Check sheet for the modelled part. Datum: model origin and axes. Units: mm. Face numbers are marked on the shaded views. Give positions to 0.01 mm unless a question says otherwise; leave off trailing zeros. Order: outer loops, then holes, each group sorted by start corner. A loop starts at its lowest first (then second) coordinate and runs counter-clockwise, first axis right, second up. Notation, with made-up numbers: (63, 40) - (85, 40) arc R7 ccw to (85, 47) - close; hole circle Ø7 at (-5, 0). An arc over 180 degrees is marked (long way). Answer in a Markdown table with one row per item.
from build123d import *

# Parameters (mm, degrees)
SKETCH1_R           = 1.75
BOSS_EXTRUDE2_DEPTH = 3
CUT_EXTRUDE5_DEPTH  = 117.344085899


with BuildPart() as part:
    # Sketch1 → Boss-Extrude2 (new body)
    # profile 1 of 6: a face of its own
    with BuildSketch(Plane.XY):
        with BuildLine():
            Line((-61.518289963, 44.547727215), (-78.684996473, 61.714433725))
            ThreePointArc((-78.684996473, 61.714433725), (-82.079566173, 51.162002537), (-75.485462345, 42.251632055))
            ThreePointArc((-75.485462345, 42.251632055), (-69.588581896, 41.003233411), (-63.818207412, 42.745208303))
            ThreePointArc((-63.818207412, 42.745208303), (-63.605961831, 42.89146595), (-63.383207651, 43.021158129))
            ThreePointArc((-63.383207651, 43.021158129), (-62.41276888, 43.738044879), (-61.518289963, 44.547727215))
        make_face()
        with Locations((-75.306872196, 51.265241636)):
            Circle(SKETCH1_R, mode=Mode.SUBTRACT)
    # profile 2 of 6: a face of its own
    with BuildSketch(Plane.XY):
        with BuildLine():
            ThreePointArc((-63.818207412, 42.745208303), (-69.588581896, 41.003233411), (-75.485462345, 42.251632055))
            ThreePointArc((-75.485462345, 42.251632055), (-66.626510988, 39.720558383), (-58.255022397, 43.568354094))
            ThreePointArc((-58.255022397, 43.568354094), (-59.291136488, 43.01863263), (-60.457290906, 43.144370333))
            ThreePointArc((-60.457290906, 43.144370333), (-61.934255267, 43.415364041), (-63.383207651, 43.021158129))
            ThreePointArc((-63.383207651, 43.021158129), (-63.599243517, 42.880875383), (-63.818207412, 42.745208303))
        make_face()
    # profile 3 of 6: a face of its own
    with BuildSketch(Plane.XY):
        with BuildLine():
            Line((-53.033008589, 53.033008589), (-61.518289963, 44.547727215))
            ThreePointArc((-61.518289963, 44.547727215), (-62.41276888, 43.738044879), (-63.383207651, 43.021158129))
            ThreePointArc((-63.383207651, 43.021158129), (-61.934255267, 43.415364041), (-60.457290906, 43.144370333))
            ThreePointArc((-60.457290906, 43.144370333), (-59.291136488, 43.01863263), (-58.255022397, 43.568354094))
            Line((-58.255022397, 43.568354094), (-50.911688245, 50.911688245))
            Line((-50.911688245, 50.911688245), (-53.033008589, 53.033008589))
        make_face()
    # profile 4 of 6: a face of its own
    with BuildSketch(Plane.XY):
        with BuildLine():
            Line((-44.547727215, 61.518289963), (-53.033008589, 53.033008589))
            Line((-53.033008589, 53.033008589), (-50.911688245, 50.911688245))
            Line((-50.911688245, 50.911688245), (-43.568354094, 58.255022397))
            ThreePointArc((-43.568354094, 58.255022397), (-43.01863263, 59.291136488), (-43.144370333, 60.457290906))
            ThreePointArc((-43.144370333, 60.457290906), (-43.415364041, 61.934255267), (-43.021158129, 63.383207651))
            ThreePointArc((-43.021158129, 63.383207651), (-43.738044879, 62.41276888), (-44.547727215, 61.518289963))
        make_face()
    # profile 5 of 6: a face of its own
    with BuildSketch(Plane.XY):
        with BuildLine():
            ThreePointArc((-42.745208303, 63.818207412), (-42.880875383, 63.599243517), (-43.021158129, 63.383207651))
            ThreePointArc((-43.021158129, 63.383207651), (-43.415364041, 61.934255267), (-43.144370333, 60.457290906))
            ThreePointArc((-43.144370333, 60.457290906), (-43.01863263, 59.291136488), (-43.568354094, 58.255022397))
            ThreePointArc((-43.568354094, 58.255022397), (-39.720558383, 66.626510988), (-42.251632055, 75.485462345))
            ThreePointArc((-42.251632055, 75.485462345), (-41.003233411, 69.588581896), (-42.745208303, 63.818207412))
        make_face()
    # profile 6 of 6: a face of its own
    with BuildSketch(Plane.XY):
        with BuildLine():
            Line((-61.714433725, 78.684996473), (-44.547727215, 61.518289963))
            ThreePointArc((-44.547727215, 61.518289963), (-43.738044879, 62.41276888), (-43.021158129, 63.383207651))
            ThreePointArc((-43.021158129, 63.383207651), (-42.89146595, 63.605961831), (-42.745208303, 63.818207412))
            ThreePointArc((-42.745208303, 63.818207412), (-41.003233411, 69.588581896), (-42.251632055, 75.485462345))
            ThreePointArc((-42.251632055, 75.485462345), (-51.162002537, 82.079566173), (-61.714433725, 78.684996473))
        make_face()
        with Locations((-51.265241636, 75.306872196)):
            Circle(SKETCH1_R, mode=Mode.SUBTRACT)
    extrude(amount=BOSS_EXTRUDE2_DEPTH)

    # Sketch2 → Cut-Extrude5 (cut, through all)
    with BuildSketch(Plane.XY.offset(3)):
        with BuildLine():
            Line((-87.146030282, 55.882108481), (-82.002155393, 50.738233593))
            ThreePointArc((-82.002155393, 50.738233593), (-81.721300187, 56.642700912), (-78.684996473, 61.714433725))
            Line((-78.684996473, 61.714433725), (-74.855475867, 57.884913119))
            Line((-74.855475867, 57.884913119), (-73.595511338, 59.144877648))
            Line((-73.595511338, 59.144877648), (-82.002155393, 67.551521704))
            Line((-82.002155393, 67.551521704), (-87.146030282, 55.882108481))
        make_face()
        with BuildLine():
            ThreePointArc((-78.684996473, 61.714433725), (-81.721300187, 56.642700912), (-82.002155393, 50.738233593))
            Line((-82.002155393, 50.738233593), (-74.855475867, 57.884913119))
            Line((-74.855475867, 57.884913119), (-78.684996473, 61.714433725))
        make_face()
        with BuildLine():
            Line((-71.077925903, 40.135754876), (-82.002155393, 50.738233593))
            ThreePointArc((-82.002155393, 50.738233593), (-79.729344323, 45.738159691), (-75.485462345, 42.251632055))
            ThreePointArc((-75.485462345, 42.251632055), (-73.379988253, 40.988939163), (-71.077925903, 40.135754876))
        make_face()
        with BuildLine():
            ThreePointArc((-75.485462345, 42.251632055), (-79.729344323, 45.738159691), (-82.002155393, 50.738233593))
            Line((-82.002155393, 50.738233593), (-82.002155393, 40.135754876))
            Line((-82.002155393, 40.135754876), (-71.077925903, 40.135754876))
            ThreePointArc((-71.077925903, 40.135754876), (-73.379988253, 40.988939163), (-75.485462345, 42.251632055))
        make_face()
        with BuildLine():
            ThreePointArc((-61.714433725, 78.684996473), (-56.642700912, 81.721300187), (-50.738233593, 82.002155393))
            Line((-50.738233593, 82.002155393), (-55.882108481, 87.146030282))
            Line((-55.882108481, 87.146030282), (-67.551521704, 82.002155393))
            Line((-67.551521704, 82.002155393), (-59.144877648, 73.595511338))
            Line((-59.144877648, 73.595511338), (-57.884913119, 74.855475867))
            Line((-57.884913119, 74.855475867), (-61.714433725, 78.684996473))
        make_face()
        with BuildLine():
            Line((-57.884913119, 74.855475867), (-50.738233593, 82.002155393))
            ThreePointArc((-50.738233593, 82.002155393), (-56.642700912, 81.721300187), (-61.714433725, 78.684996473))
            Line((-61.714433725, 78.684996473), (-57.884913119, 74.855475867))
        make_face()
        with BuildLine():
            ThreePointArc((-42.251632055, 75.485462345), (-45.738159691, 79.729344323), (-50.738233593, 82.002155393))
            Line((-50.738233593, 82.002155393), (-40.135754876, 71.077925903))
            ThreePointArc((-40.135754876, 71.077925903), (-40.988939163, 73.379988253), (-42.251632055, 75.485462345))
        make_face()
        with BuildLine():
            Line((-40.135754876, 82.002155393), (-50.738233593, 82.002155393))
            ThreePointArc((-50.738233593, 82.002155393), (-45.738159691, 79.729344323), (-42.251632055, 75.485462345))
            ThreePointArc((-42.251632055, 75.485462345), (-40.988939163, 73.379988253), (-40.135754876, 71.077925903))
            Line((-40.135754876, 71.077925903), (-40.135754876, 82.002155393))
        make_face()
    extrude(amount=-CUT_EXTRUDE5_DEPTH, mode=Mode.SUBTRACT)


solid = part.part
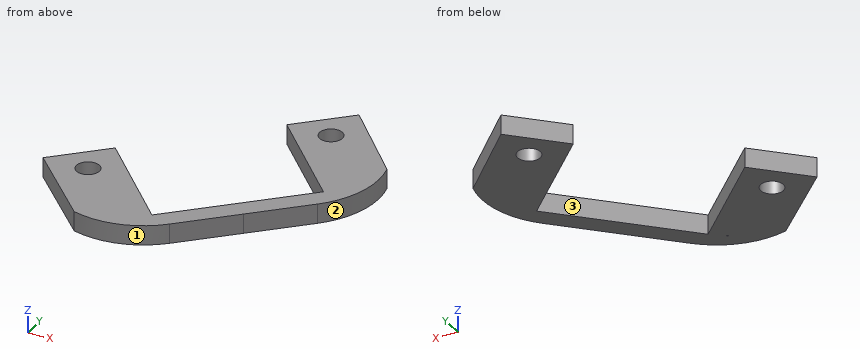
(1) Cross-section at C-C, the plane y = 76.5. Record the cut outline in (x, z), then the cut area to 3 significant figures.
Geometry says:
| item | result |
|---|---|
| outline | (-56.24, 0) - (-52.55, 0) - (-52.55, 3) - (-56.24, 3) - close; (-49.99, 0) - (-45.4, 0) - (-45.4, 3) - (-49.99, 3) - close |
| area | 24.8 mm² |
(2) Cross-section at B-B, the plane y = 50. Record the cut outline in (x, z), then the cut area to 3 significant figures.
Geometry says:
| item | result |
|---|---|
| outline | (-81.24, 0) - (-76.52, 0) - (-76.52, 3) - (-81.24, 3) - close; (-74.1, 0) - (-66.97, 0) - (-66.97, 3) - (-74.1, 3) - close; (-56.07, 0) - (-51.82, 0) - (-51.82, 3) - (-56.07, 3) - close |
| area | 48.3 mm² |
(3) Cross-section at A-A, the plane x = -56. Record the cut outline in (y, z), then the cut area to 3 significant figures.
Geometry says:
| item | result |
|---|---|
| outline | (45.82, 0) - (50.07, 0) - (50.07, 3) - (45.82, 3) - close; (72.97, 0) - (76.74, 0) - (76.74, 3) - (72.97, 3) - close |
| area | 24.0 mm² |
(4) Mould release check, pull along X, two halves, no side actions. Record for the marked faces 1, 2 and 3: pulls with the +X half, pulls with the -X half, needs draft (parallel to the pull), parting line crosses it, or undercut.
Geometry says:
| item | result |
|---|---|
| face 1 | parting line crosses it |
| face 2 | pulls with the +X half |
| face 3 | undercut |
(5) Gauge pin test, flat end, axial feed: P1, Ø5, axis at x = -48.5, y = 56.5, coming from the -Z side. Record the tip position at first contact, or that the pin passes through.
Geometry says:
| item | result |
|---|---|
| P1 | z = 0 |
(6) Cross-section at D-D, the plane z = 1.7. Record the cut outline in (x, y).
Geometry says:
| item | result |
|---|---|
| outline | (-82, 50.74) - (-71.08, 40.14) arc R13.27 ccw to (-58.26, 43.57) - (-43.57, 58.26) arc R13.27 ccw to (-40.14, 71.08) - (-50.74, 82) - (-57.88, 74.86) - (-44.55, 61.52) - (-61.52, 44.55) - (-74.86, 57.88) - close; hole circle Ø3.5 at (-75.31, 51.27); hole (-63.82, 42.75) arc R12.14 ccw to (-63.38, 43.02) arc R3.39 ccw to start; hole circle Ø3.5 at (-51.27, 75.31); hole (-43.02, 63.38) arc R12.14 ccw to (-42.75, 63.82) arc R3.39 ccw to start |
(7) Thickness scan on L1, parallel to Y at x = -50, z = 1.5; L2, parallel to X at y = 51, z = 1.4; L3, parallel to X at y = 54, z = 1.5. Record the ranges inside material, lowest first.
Geometry says:
| item | result |
|---|---|
| L1 | 51.82 to 56.07, 66.97 to 74.1, 76.52 to 81.24 |
| L2 | -81.74 to -77.04, -73.58 to -67.97, -55.07 to -50.82 |
| L3 | -78.74 to -70.97, -52.07 to -47.82 |
